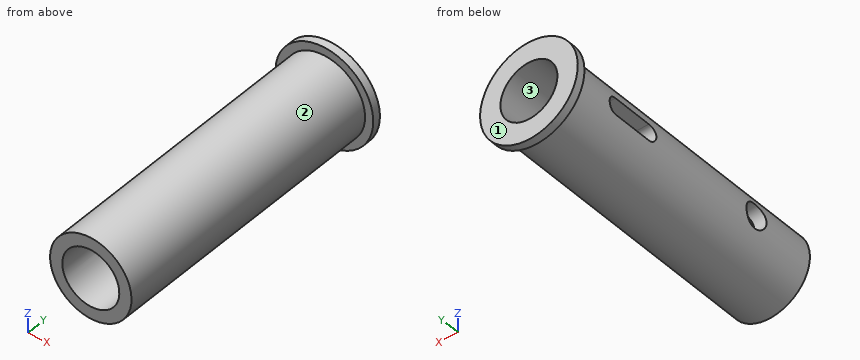
```python
from build123d import *

# Parameters (mm, degrees)
SKETCH4_R               = 10
BOSS_EXTRUDE2_DEPTH     = 70
SKETCH5_R               = 12
BOSS_EXTRUDE3_DEPTH     = 2
CUT_EXTRUDE1_REACH      = 75.973
SKETCH6_R               = 7
CUT_EXTRUDE3_REACH      = 75.973
CUT_EXTRUDE3_END_RADIUS = 10
SKETCH7_R               = 3
CUT_EXTRUDE5_DEPTH      = 1
CUT_EXTRUDE5_DEPTH_BACK = 74.972968133
SKETCH7_4_R             = 2


with BuildPart() as part:
    # Sketch4 → Boss-Extrude2 (new body)
    with BuildSketch(Plane(origin=(0, 0, 0), x_dir=(1, 0, 0), z_dir=(0, 1, 0))):
        with Locations(Location((0, 0, 0), (0, 0, 270))):
            Circle(SKETCH4_R)
    extrude(amount=BOSS_EXTRUDE2_DEPTH)

    # Sketch5 → Boss-Extrude3 (add)
    with BuildSketch(Plane(origin=(0, 70, 0), x_dir=(1, 0, 0), z_dir=(0, 1, 0))):
        with Locations(Location((0, 0, 0), (0, 0, 270))):
            Circle(SKETCH5_R)
    extrude(amount=BOSS_EXTRUDE3_DEPTH)

    # Sketch6 → Cut-Extrude1 (cut, up to next)
    with BuildSketch(Plane.XZ, mode=Mode.PRIVATE) as cut_extrude1_sk1:
        with Locations(Location((0, 0, 0), (0, 0, 270))):
            Circle(SKETCH6_R)
    cut_extrude1_tool1 = extrude(cut_extrude1_sk1.sketch, amount=-CUT_EXTRUDE1_REACH, mode=Mode.PRIVATE) & part.part
    add(cut_extrude1_tool1.solids().sort_by_distance((0, 0, 0))[0], mode=Mode.SUBTRACT)

    # Cut-Extrude3: up to this cylinder (the profile starts inside it)
    cut_extrude3_end = Plane(origin=(0, 16, 0), z_dir=(0, -1, 0)) * Cylinder(CUT_EXTRUDE3_END_RADIUS, 172.946, mode=Mode.PRIVATE)
    # Sketch7 → Cut-Extrude3 (cut, up to the surface)
    with BuildSketch(Plane(origin=(0, 0, 0), x_dir=(0, 0, -1), z_dir=(1, 0, 0)), mode=Mode.PRIVATE) as cut_extrude3_sk1:
        with Locations((0, 16)):
            Circle(SKETCH7_R)
    cut_extrude3_tool1 = extrude(cut_extrude3_sk1.sketch, amount=-CUT_EXTRUDE3_REACH, mode=Mode.PRIVATE) & cut_extrude3_end
    add(cut_extrude3_tool1.solids().sort_by_distance((0, 16, 0))[0], mode=Mode.SUBTRACT)

    # Sketch7<4> → Cut-Extrude5 (cut, two sides: drawn at the far end of the back side and taken through both)
    with BuildSketch(Plane(origin=(0, 0, 0), x_dir=(0, 0, -1), z_dir=(1, 0, 0)).offset(-CUT_EXTRUDE5_DEPTH_BACK)):
        with BuildLine():
            Line((2, 53), (2, 58))
            ThreePointArc((2, 58), (0, 60), (-2, 58))
            Line((-2, 58), (-2, 53))
            ThreePointArc((-2, 53), (0, 55), (2, 53))
        make_face()
        with Locations((0, 53)):
            Circle(SKETCH7_4_R)
        with BuildLine():
            Line((2, 48), (2, 53))
            ThreePointArc((2, 53), (0, 51), (-2, 53))
            Line((-2, 53), (-2, 48))
            ThreePointArc((-2, 48), (0, 46), (2, 48))
        make_face()
    extrude(amount=CUT_EXTRUDE5_DEPTH + CUT_EXTRUDE5_DEPTH_BACK, mode=Mode.SUBTRACT)


solid = part.part
```
For this review, take the finished solid that the model builds, in its own axes (mm). Face numbers are marked on the shaded views. Round coordinates to 2 decimals unless told otherwise and drop trailing zeros. Write each loop counter-clockwise with the first axis right and the second up, starting at its lowest first coordinate (ties: lowest second). Pieces come first, ordered by that corner, then holes. Notation, with made-up numbers: M -25.5,52.25 L 2.5,52.25 A17 ccw 2.5,85.25 Z; hole C 57,68 d6. An arc over 180 degrees is marked long. One line per item, written item: value. Start each with the question number.
(1) Wall thickness on line 1 (Y direction, x = -7.5, z = 0); line 2 (X direction, y = 30, z = 0); line 3 (X direction, y = 16, z = 0): over which ranges is each line inside the solid? List them lowest first.
(2) We need section C-C (z = -5.75). Give the boundary of the cut face in (x, y).
(3) We need section D-D (y = 8.5). Give the boundary of the cut face in (x, z), and give its area (3 significant figures).
(4) Insertion check: pin 1 (2.5 mm diameter, centred on x = -8.5, y = 54, fed in from -Z); pin 2 (5 mm diameter, centred on x = -7.5, y = 17, fed in from -Z); pin 3 (2.5 mm diameter, centred on x = -9, y = 55.5, fed in from +Z); pin 4 (4 mm diameter, centred on x = 3, z = 3, fed in from +Y). Each pin has a flat end and moves straight along its axis. Give the tip position at first contact, or say it passes through.
(5) We need section A-A (z = 0). Give the boundary of the cut face in (x, y).
(6) The part is to be moulded in two halves that separate along X. For the marked faces 1, 2 and 3, say which applies: released by +X, released by -X, zero draft, split by the parting line, or undercut.
(7) We need section B-B (x = 0). Give the boundary of the cut face in (y, z), and give its area (3 significant figures).
Result:
1. line 1: 0 to 13, 19 to 46, 60 to 72
1. line 2: -10 to -7, 7 to 10
1. line 3: 7 to 10
2. outline: M -10.53,70 L -8.18,70 L -8.18,0 L -3.99,0 L -3.99,72 L -10.53,72 Z; M 3.99,0 L 8.18,0 L 8.18,70 L 10.53,70 L 10.53,72 L 3.99,72 Z
3. outline: C 0,0 d20; hole C 0,0 d14
3. area: 160 mm²
4. pin 1: z = -6.89
4. pin 2: z = -8.66
4. pin 3: z = 6.32
4. pin 4: through
5. outline: M -12,70 L -10,70 L -10,60 L -7,60 L -7,72 L -12,72 Z; M -10,0 L -7,0 L -7,13 L -10,13 Z; M -10,19 L -7,19 L -7,46 L -10,46 Z; M 7,0 L 10,0 L 10,70 L 12,70 L 12,72 L 7,72 Z
6. face 1: zero draft
6. face 2: split by the parting line
6. face 3: undercut
7. outline: M 0,-10 L 70,-10 L 70,-12 L 72,-12 L 72,-7 L 0,-7 Z; M 0,7 L 72,7 L 72,12 L 70,12 L 70,10 L 0,10 Z
7. area: 440 mm²
